from build123d import *

# Parameters (mm, degrees)
SKETCH_1_W          = 13
SKETCH_1_H          = 80
SKETCH_1_R          = 2.1
SKETCH_1_R_2        = 1.65
EXTRUDE_1_DEPTH     = 13
CUT_EXTRUDE_4_DEPTH = 13
CUT_EXTRUDE_5_DEPTH = 3


with BuildPart() as part:
    # 草图1 → 凸台-拉伸1 (new body)
    with BuildSketch(Plane.XY):
        with Locations((0.560222304, -25.704710145)):
            Rectangle(SKETCH_1_W, SKETCH_1_H)
        with Locations((0.560222304, 9.295289855)):
            Circle(SKETCH_1_R, mode=Mode.SUBTRACT)
        with Locations((0.560222304, -5.704710145)):
            Circle(SKETCH_1_R, mode=Mode.SUBTRACT)
        with Locations((0.560222304, -60.704710145)):
            Circle(SKETCH_1_R_2, mode=Mode.SUBTRACT)
        with Locations((0.560222304, -45.704710145)):
            Circle(SKETCH_1_R_2, mode=Mode.SUBTRACT)
    extrude(amount=EXTRUDE_1_DEPTH)

    # 草图4 → 切除-拉伸4 (cut)
    with BuildSketch(Plane(origin=(7.060222304, 0, 0), x_dir=(0, 0, -1), z_dir=(1, 0, 0))):
        with BuildLine():
            ThreePointArc((-4.438447187, -25.704710145), (-6.5, -17.204710145), (-8.561552813, -25.704710145))
            ThreePointArc((-8.561552813, -25.704710145), (-6.5, -34.204710145), (-4.438447187, -25.704710145))
        make_face()
    extrude(amount=-CUT_EXTRUDE_4_DEPTH, mode=Mode.SUBTRACT)

    # 草图5 → 切除-拉伸5 (cut)
    with BuildSketch(Plane.XZ.offset(65.704710145)):
        Polygon((0, 10.380755621), (-2.765074416, 7.090643354), (-0.798384611, 7.090643354), (-0.798384611, 1.381735054), (0.79750081, 1.381735054), (0.79750081, 7.090643354), (2.925348038, 7.090643354), align=None)
    extrude(amount=-CUT_EXTRUDE_5_DEPTH, mode=Mode.SUBTRACT)


solid = part.part
Check sheet for the modelled part. Datum: model origin and axes. Units: mm. A direction names the side the tool comes from. Round coordinates to 2 decimals unless told otherwise and drop trailing zeros. Write each loop counter-clockwise with the first axis right and the second up, starting at its lowest first coordinate (ties: lowest second). Pieces come first, ordered by that corner, then holes. Notation, with made-up numbers: (-36, -2.75) - (22, -2.75) arc R6 cw to (22, 5.25) - close; hole circle Ø3 at (34.5, 49). An arc over 180 degrees is marked (long way). Return JSON: item names as keys, results as strings.
Q1. Draft check along Y on faces 3 (the flat face through (0, 14.295, 6)), 4 (the cylindrical face through (2.56, -5.07, 6.41)), 5 (the cylindrical face through (0.651, -17.208, 6.332)), 6 (the flat face through (0, -25, 13)). Enter one of: released by +Y, released by -Y, zero draft, split by the parting line, or undercut.
Returned:
{"face 3": "released by +Y", "face 4": "undercut", "face 5": "undercut", "face 6": "zero draft"}
Q2. Cross-section at B-B (y = -27). Record the boundary of the cut face in (x, z).
Returned:
{"outline": "(-5.94, 0) - (7.06, 0) - (7.06, 2.9) - (-5.94, 2.9) - close; (-5.94, 10.1) - (7.06, 10.1) - (7.06, 13) - (-5.94, 13) - close"}
Q3. Scan lines: L1, parallel to Y at x = 4, z = 6.25; L2, parallel to Y at x = 2, z = 1.5; L3, parallel to X at y = -7, z = 2.5. Record each from-to range of solid material in increasing order. Write a range as from..to.
Returned:
{"L1": "y = -65.7..-34.2, -17.21..14.3", "L2": "y = -65.7..-61.51, -59.9..-46.51, -44.9..-7.23, -4.18..7.77, 10.82..14.3", "L3": "x = -5.94..-1.09, 2.21..7.06"}
Q4. Cross-section at C-C (x = 4.75). Record the boundary of the cut face in (y, z), then the cut area to 3 significant figures.
Returned:
{"outline": "(-65.7, 0) - (14.3, 0) - (14.3, 13) - (-65.7, 13) - close; hole (-25.7, 4.44) arc R4.5 ccw (long way) to (-25.7, 8.56) arc R4.5 ccw (long way) to start", "area": "916 mm²"}
Q5. Cross-section at A-A (z = 9.5). Record the boundary of the cut face in (x, y), then the cut area to 3 significant figures.
Returned:
{"outline": "(-5.94, -65.7) - (-0.74, -65.7) - (-0.74, -62.7) - (0.78, -62.7) - (0.78, -65.7) - (7.06, -65.7) - (7.06, -33.06) - (-5.94, -33.06) - close; (-5.94, -26.35) - (7.06, -26.35) - (7.06, -25.06) - (-5.94, -25.06) - close; (-5.94, -18.35) - (7.06, -18.35) - (7.06, 14.3) - (-5.94, 14.3) - close; hole circle Ø4.2 at (0.56, -5.7); hole circle Ø4.2 at (0.56, 9.3); hole circle Ø3.3 at (0.56, -60.7); hole circle Ø3.3 at (0.56, -45.7)", "area": "816 mm²"}
Q6. Depth check by flat-ended pin: P1, Ø4, axis at x = 0.56, y = -5.7, coming from the -Z side. Enter the tip coordinate at first touch or a pass-through.
Returned:
{"P1": "passes through"}
Q7. Access from +Z, -Z, +X, -X, +Y, -Y to the whole of each face (thin tool, end or side, straight path). Record for faces 1 (the cylindrical face through (1.32, -62.17, 6.41)), 2 (the flat face through (1.483, -64.226, 8.713)).
Returned:
{"face 1": "+Z, -Z", "face 2": "-Y"}
